Can you work these out from the model? Positions are in its coordinate system, mm. Give positions to 0.01 mm unless a question says otherwise; leave off trailing zeros. Order: outer loops, then holes, each group sorted by start corner. A loop starts at its lowest first (then second) coordinate and runs counter-clockwise, first axis right, second up. Notation, with made-up numbers: (-28, 16.5) - (-4, 16.5) arc R26 ccw to (-4, 42.5) - close; hole circle Ø10 at (76, -11.5). An arc over 180 degrees is marked (long way). Return JSON: item names as keys, results as strings.
Autodesk Inventor part; units mm, degrees
ref_plane "YZ Plane" through (0, 0, 0) normal (1, 0, 0) x (0, 1, 0)
ref_plane "XZ Plane" through (0, 0, 0) normal (0, 1, 0) x (-1, 0, 0)
ref_plane "XY Plane" through (0, 0, 0) normal (0, 0, 1) x (1, 0, 0)
sketch "Skizze1" plane through (0, 0, 0) normal (0, 1, 0) x (-1, 0, 0)
  circle A0 centre (0, 0) radius 7.5
  circle A1 centre (7.5, 0) radius 1.5
  circle A2 centre (-7.5, 0) radius 1.5
  dimension "d0" = 15
  dimension "d1" = 3
  dimension "d2" = 3
extrude "Extrusion1" add sketch "Skizze1" along normal blind 12 contours A0 A1 | A1 A0 A2 | A2 A0 picked at (7.0094, -0.2882) picked at (-6.9889, 0)
sketch "Skizze2" plane through (0, 0, 0) normal (0, -1, 0) x (1, 0, 0)
  circle A0 centre (0, 0) radius 7.5
  circle A1 centre (7.5, 0) radius 1.5
  circle A2 centre (-7.5, 0) radius 1.5
  dimension "d5" = 3
  dimension "d6" = 3
extrude "Extrusion2" add sketch "Skizze2" against normal blind 8 contours A0 A1 | A0 A1 | A2 A0 | A0 A2
chamfer "Fase1" distance 2 angle 45 1 edges at (7.5, 12, 0)
fillet "Rundung1" radius 1 2 edges at (7.5, 10, 0) (5.5, 12, 0)
fillet "Rundung2" radius 0.5 2 edges at (9, 8, 0) (-9, 8, 0)
properties part number "case"
1. If I drill on L1, parallel to Z at x = -7.5, y = 4; L2, parallel to Z at x = -1.5, y = 7.25; L3, parallel to X at y = 10.5, z = 1.5, over which ranges is the centre line in solid material (lowest first)? Write a range as [from, to].
Checks:
{"L1": "[-1.5, 1.5]", "L2": "[-7.35, 7.35]", "L3": "[-6.84, 6.84]"}
2. Suppose I cut it at A-A (y = 6.25). List the corners of the cut face in (x, z) for me, plus the area to 3 significant figures.
Checks:
{"outline": "(-7.35, -1.49) arc R7.5 ccw to (7.35, -1.49) arc R1.5 ccw (long way) to (7.35, 1.49) arc R7.5 ccw to (-7.35, 1.49) arc R1.5 ccw (long way) to start", "area": "184 mm^2"}
3. For pin 1 Ø0.9 at (x, z) = (-8, 0) entering from +Y; pin 2 Ø6 at (y, z) = (8.5, 2) entering from -X; pin 3 Ø3 at (y, z) = (9.5, 2.5) entering from +X; pin 4 Ø3 at (x, y) = (-6.5, 3) entering from -Z, each with a flat end and sliding along its axis, tell me the tip position at first contact or that it passes through.
Checks:
{"pin 1": "y = 8", "pin 2": "x = -9", "pin 3": "x = 7.43", "pin 4": "z = -5.59"}
